Study the drawing (mm; zero at the part's minimum x, y, z) and answer. Coordinates: 2 decimals unless noted, no trailing zeros. Write each loop counter-clockwise with the first axis right and the second up, starting at its lowest first coordinate (ties: lowest second). Pieces come first, ordered by that corner, then holes. Notation, with made-up numbers: M 63,-30.75 L 77,-30.75 A20 ccw 77,-13.75 Z; hole C -31.5,0 d5. An arc over 180 degrees is marked long. Answer as a JSON object with one key per item and string values. Group by question number.
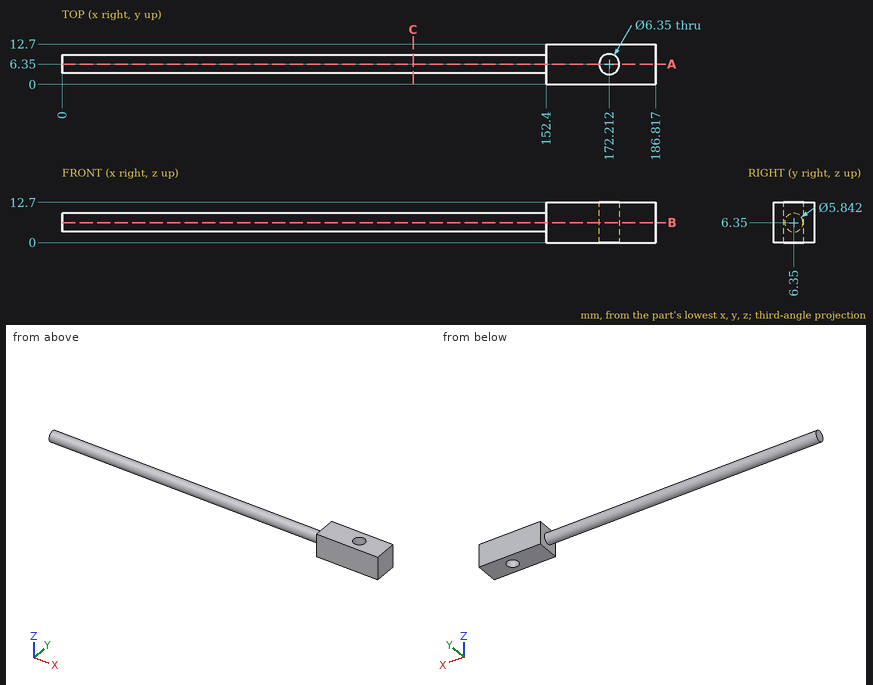
Item 1: A cutting plane is placed at A-A, the plane y = 6.35. Write down the section's boundary in (x, z), and give its area (3 significant figures).
Item 2: A cutting plane is placed at C-C, the plane x = 110.5. Write down the section's boundary in (y, z).
Item 3: Consider L1, parallel to Z at x = 18.5, y = 6; L2, parallel to X at y = 11.25, z = 11.25; L3, parallel to X at y = 4.5, z = 1. Determine where each line is inside the solid, lowest interval first. Write a range as from..to.
Item 4: A cutting plane is placed at B-B, the plane z = 6.35. Write down the section's boundary in (x, y) (3 decimals).
Item 5: Flat-ended cylindrical pins translate along their axes: pin 1 Ø3 at (x, z) = (36, 4.5) entering from -Y; pin 2 Ø2 at (x, y) = (99, 6) entering from +Z; pin 3 Ø7.5 at (x, y) = (172.212, 6.35) entering from +Z; pin 4 Ø4 at (x, y) = (129.5, 9) entering from -Z. Find the tip coordinate at first contact, or state that the pin passes through.
Answer:
{
 "1": {"outline": "M 0,3.43 L 152.4,3.43 L 152.4,0 L 169.04,0 L 169.04,12.7 L 152.4,12.7 L 152.4,9.27 L 0,9.27 Z; M 175.39,0 L 186.82,0 L 186.82,12.7 L 175.39,12.7 Z", "area": "1,250 mm2"},
 "2": {"outline": "C 6.35,6.35 d5.84"},
 "3": {"L1": "3.45..9.25", "L2": "152.4..186.82", "L3": "152.4..169.63, 174.79..186.82"},
 "4": {"outline": "M 0,3.429 L 152.4,3.429 L 152.4,0 L 186.817,0 L 186.817,12.7 L 152.4,12.7 L 152.4,9.271 L 0,9.271 Z; hole C 172.212,6.35 d6.35"},
 "5": {"pin 1": "y = 3.45", "pin 2": "z = 9.27", "pin 3": "z = 12.7", "pin 4": "z = 3.5"}
}
